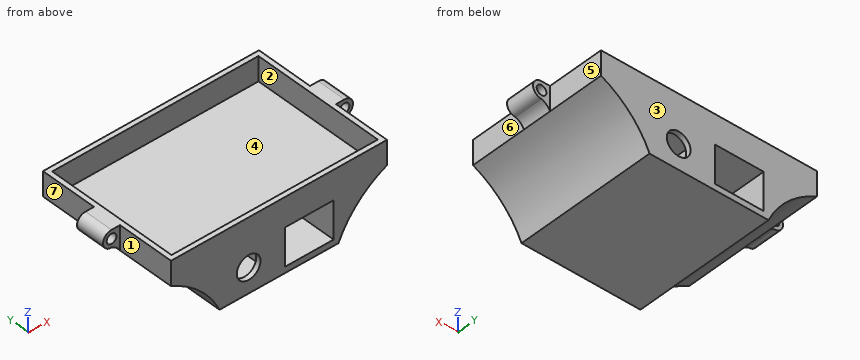
from build123d import *

# Parameters (mm, degrees)
F1_DEPTH       = 29.5
F1_DEPTH_BACK  = 29.5
F2_R           = 2
F3_DEPTH       = 6
F3_DEPTH_BACK  = 6
F4_W           = 85
F4_H           = 55
F5_DEPTH       = 10
F6_W           = 20
F6_H           = 15.5
F7_DEPTH       = 29.5
F7_DEPTH_BACK  = 27.5
F8_W           = 20
F8_H           = 15.5
F9_DEPTH       = 57
F10_R          = 4.9
F11_DEPTH      = 80
F11_DEPTH_BACK = 80


with BuildPart() as f1:
    # F0 (on Front) → F1 (new body, two sides)
    with BuildSketch(Plane.XZ) as f1_sk:
        with BuildLine():
            Line((44.5, 15), (-44.5, 15))
            Line((-44.5, 15), (-44.5, 5))
            ThreePointArc((-44.5, 5), (-32.6732418632, -3.1732418632), (-24.5, -15))
            Line((-24.5, -15), (0, -15))
            Line((0, -15), (24.5, -15))
            ThreePointArc((24.5, -15), (32.6732418632, -3.1732418632), (44.5, 5))
            Line((44.5, 5), (44.5, 15))
        make_face()
    extrude(amount=F1_DEPTH)
    extrude(f1_sk.sketch, amount=-F1_DEPTH_BACK)

    # F2 (on Front) → F3 (join, two sides)
    with BuildSketch(Plane.XZ) as f3_sk:
        with BuildLine():
            Line((48, 15), (44.5, 15))
            Line((44.5, 15), (44.5, 5))
            ThreePointArc((44.5, 5), (45.9503951439, 6.8495389988), (48, 8))
            ThreePointArc((48, 8), (51.5, 11.5), (48, 15))
        make_face()
        with Locations((48, 11.5)):
            Circle(F2_R, mode=Mode.SUBTRACT)
        with BuildLine():
            Line((-44.5, 5), (-44.5, 15))
            Line((-44.5, 15), (-48, 15))
            ThreePointArc((-48, 15), (-51.5, 11.5), (-48, 8))
            ThreePointArc((-48, 8), (-45.9503951439, 6.8495389988), (-44.5, 5))
        make_face()
        with Locations((-48, 11.5)):
            Circle(F2_R, mode=Mode.SUBTRACT)
    extrude(amount=F3_DEPTH)
    extrude(f3_sk.sketch, amount=-F3_DEPTH_BACK)

    # F4 (on face) → F5 (cut)
    with BuildSketch(Plane.XY.offset(15)):
        Rectangle(F4_W, F4_H)
    extrude(amount=-F5_DEPTH, mode=Mode.SUBTRACT)

    # F6 (on Front) → F7 (cut, two sides)
    with BuildSketch(Plane.XZ) as f7_sk:
        with Locations((-12.5, -4.75)):
            Rectangle(F6_W, F6_H)
    extrude(amount=-F7_DEPTH, mode=Mode.SUBTRACT)
    extrude(f7_sk.sketch, amount=F7_DEPTH_BACK, mode=Mode.SUBTRACT)

    # F8 (on face) → F9 (cut)
    with BuildSketch(Plane.XZ.offset(29.5)):
        with Locations((12.5, -4.75)):
            Rectangle(F8_W, F8_H)
    extrude(amount=-F9_DEPTH, mode=Mode.SUBTRACT)

    # F10 (on Front) → F11 (cut, two sides)
    with BuildSketch(Plane.XZ) as f11_sk:
        with Locations((-12.5, -4.75)):
            Circle(F10_R)
        with Locations((12.5, -4.75)):
            Circle(F10_R)
    extrude(amount=-F11_DEPTH, mode=Mode.SUBTRACT)
    extrude(f11_sk.sketch, amount=F11_DEPTH_BACK, mode=Mode.SUBTRACT)


solid = f1.part
Could you check a few things on this model? Use its own coordinates, in mm. Face numbers are marked on the shaded views. A direction names the side the tool comes from. Coordinates: 2 decimals unless noted, no trailing zeros. Order: outer loops, then holes, each group sorted by start corner. A loop starts at its lowest first (then second) coordinate and runs counter-clockwise, first axis right, second up.
Q1. Thinking about a two-plate mould opening in Y: for the marked faces 1, 2 and 3, which applies, released by +Y, released by -Y, zero draft, split by the parting line, or undercut?
Q2. Which directions (+Z, -Z, +X, -X, +Y, -Y) give clear straight access to the entire face, cutting with the end or side of a thin tool? Please do the marked faces 4, 5, 6 and 7.
Q3. Suppose I cut it at B-B on y = -1.5. Please give me the cut outline in (x, z).
Q4. Please list where these lines run through material, in increasing order: L1, parallel to Y at x = -10, z = 12.5; L2, parallel to Z at x = -19.5, y = -16; L3, parallel to X at y = -19, z = 8.
Q5. Suppose I cut it at D-D on x = 6. Please give me the cut outline in (y, z), and give its area (4 significant figures).
Q6. Suppose I cut it at A-A on z = 11.5. Please give me the cut outline in (x, y).
Q7. Suppose I cut it at C-C on y = 8. Please give me the cut outline in (x, z).
Q8. Will these pins go through, and if not, where does the flat tip stop? pin 1 (6 mm diameter, centred on x = 12.5, z = -4.75, fed in from -Y); pin 2 (6 mm diameter, centred on y = -22, z = 1.5, fed in from +X); pin 3 (10 mm diameter, centred on x = 11, y = -6, fed in from +Z); pin 4 (4.5 mm diameter, centred on x = 48, z = 11.5, fed in from -Y).
Answer:
1. face 1: zero draft
1. face 2: undercut
1. face 3: released by +Y
2. face 4: +Z
2. face 5: +Z, -Z, +X, +Y
2. face 6: +Z, -Z, +X, -Y
2. face 7: +Z, -Z, -X, +Y
3. outline: (-48, 8) arc R6 cw to (-44.5, 5) arc R40 cw to (-24.5, -15) - (24.5, -15) arc R40 cw to (44.5, 5) arc R6 cw to (48, 8) arc R3.5 ccw to (48, 15) - (42.5, 15) - (42.5, 5) - (-42.5, 5) - (-42.5, 15) - (-48, 15) arc R3.5 ccw to start; hole circle Ø4 at (-48, 11.5); hole (-22.5, -12.5) - (-2.5, -12.5) - (-2.5, 3) - (-22.5, 3) - close; hole (2.5, -12.5) - (22.5, -12.5) - (22.5, 3) - (2.5, 3) - close; hole circle Ø4 at (48, 11.5)
4. L1: y = -29.5 to -27.5, 27.5 to 29.5
4. L2: z = -15 to -12.5, 3 to 5
4. L3: x = -44.5 to -42.5, 42.5 to 44.5
5. outline: (-29.5, -15) - (29.5, -15) - (29.5, 15) - (27.5, 15) - (27.5, 5) - (-27.5, 5) - (-27.5, 15) - (-29.5, 15) - (-29.5, 3) - (27.5, 3) - (27.5, -12.5) - (-29.5, -12.5) - close
5. area: 336.5 mm2
6. outline: (-51.5, -6) - (-50, -6) - (-50, 6) - (-51.5, 6) - close; (-46, -6) - (-44.5, -6) - (-44.5, -29.5) - (44.5, -29.5) - (44.5, -6) - (46, -6) - (46, 6) - (44.5, 6) - (44.5, 29.5) - (-44.5, 29.5) - (-44.5, 6) - (-46, 6) - close; (50, -6) - (51.5, -6) - (51.5, 6) - (50, 6) - close; hole (-42.5, -27.5) - (42.5, -27.5) - (42.5, 27.5) - (-42.5, 27.5) - close
7. outline: (-44.5, 5) arc R40 cw to (-24.5, -15) - (24.5, -15) arc R40 cw to (44.5, 5) - (44.5, 15) - (42.5, 15) - (42.5, 5) - (-42.5, 5) - (-42.5, 15) - (-44.5, 15) - close; hole (-22.5, -12.5) - (-2.5, -12.5) - (-2.5, 3) - (-22.5, 3) - close; hole (2.5, -12.5) - (22.5, -12.5) - (22.5, 3) - (2.5, 3) - close
8. pin 1: passes through
8. pin 2: stops at x = 43.43
8. pin 3: stops at z = 5
8. pin 4: stops at y = -6
